Check sheet for the drawn part. Datum: minimum x, y, z corner. Units: mm. A direction names the side the tool comes from. Coordinates: 2 decimals unless noted, no trailing zeros. Order: outer loops, then holes, each group sorted by start corner. A loop starts at its lowest first (then second) coordinate and runs counter-clockwise, first axis right, second up. Notation, with made-up numbers: M -4,-35.5 L 39,-35.5 A15 ccw 39,-28.5 Z; hole C -5,55.25 d10. An arc over 180 degrees is marked long. Answer in a Markdown table with one row per item. Add a question column.
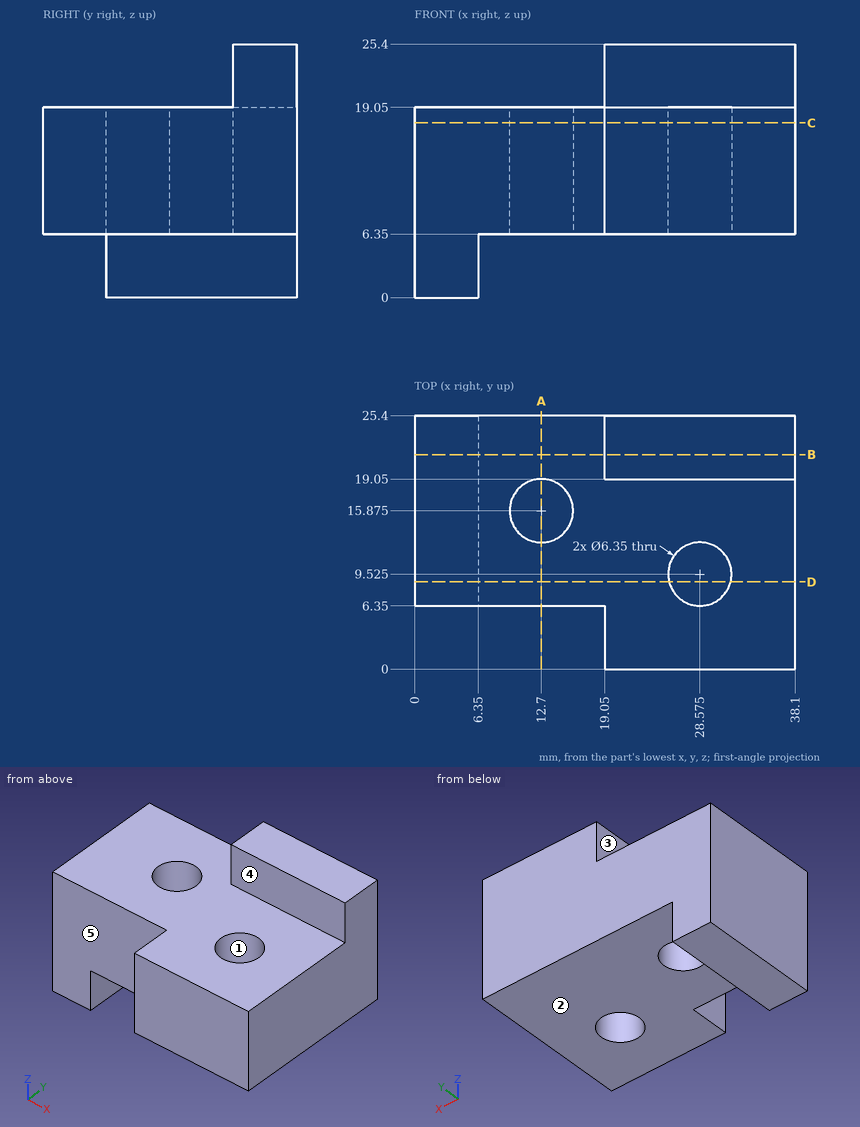
1. Section check A-A on x = 12.7. Enter the section's corners in (y, z).
2. Section check D-D on y = 8.75. Enter the section's corners in (x, z), then the cut area to 3 significant figures.
3. Section check B-B on y = 21.5. Enter the section's corners in (x, z).
4. Section check C-C on z = 17.5. Enter the section's corners in (x, y) (3 decimals), then the cut area to 3 significant figures.
5. Scan lines: line 1 (Y direction, x = 12.7, z = 16); line 2 (Z direction, x = 3, y = 18.25); line 3 (Z direction, x = 7, y = 23.5). Record each from-to range of solid material in increasing order.
6. Go/stop test with flat-tipped pins: pin 1 Ø15 at (x, z) = (5, 11.5) entering from -Y; pin 2 Ø6 at (x, y) = (19, 8) entering from -Z; pin 3 Ø1.9 at (y, z) = (5, 13) entering from -X. Record where each tip stops, or that it passes through.
7. Set-up check for the marked faces 1, 2, 3, 4 and 5: record each of +Z, -Z, +X, -X, +Y, -Y from which the full face is reachable in a straight line by a thin tool's end or side.
Result sheet:
| question | item | result |
|---|---|---|
| 1 | outline | M 6.35,6.35 L 12.7,6.35 L 12.7,19.05 L 6.35,19.05 Z; M 19.05,6.35 L 25.4,6.35 L 25.4,19.05 L 19.05,19.05 Z |
| 2 | outline | M 0,0 L 6.35,0 L 6.35,6.35 L 25.5,6.35 L 25.5,19.05 L 0,19.05 Z; M 31.65,6.35 L 38.1,6.35 L 38.1,19.05 L 31.65,19.05 Z |
| 2 | area | 446 mm^2 |
| 3 | outline | M 0,0 L 6.35,0 L 6.35,6.35 L 38.1,6.35 L 38.1,25.4 L 19.05,25.4 L 19.05,19.05 L 0,19.05 Z |
| 4 | outline | M 0,6.35 L 19.05,6.35 L 19.05,0 L 38.1,0 L 38.1,25.4 L 0,25.4 Z; hole C 12.7,15.875 d6.35; hole C 28.575,9.525 d6.35 |
| 4 | area | 783 mm^2 |
| 5 | line 1 | 6.35 to 12.7, 19.05 to 25.4 |
| 5 | line 2 | 0 to 19.05 |
| 5 | line 3 | 6.35 to 19.05 |
| 6 | pin 1 | y = 6.35 |
| 6 | pin 2 | z = 6.35 |
| 6 | pin 3 | x = 19.05 |
| 7 | face 1 | +Z, -Z |
| 7 | face 2 | -Z, +X, +Y, -Y |
| 7 | face 3 | +Z, -X, +Y, -Y |
| 7 | face 4 | +Z, +X, -X, -Y |
| 7 | face 5 | +Z, -Z, -X, -Y |
